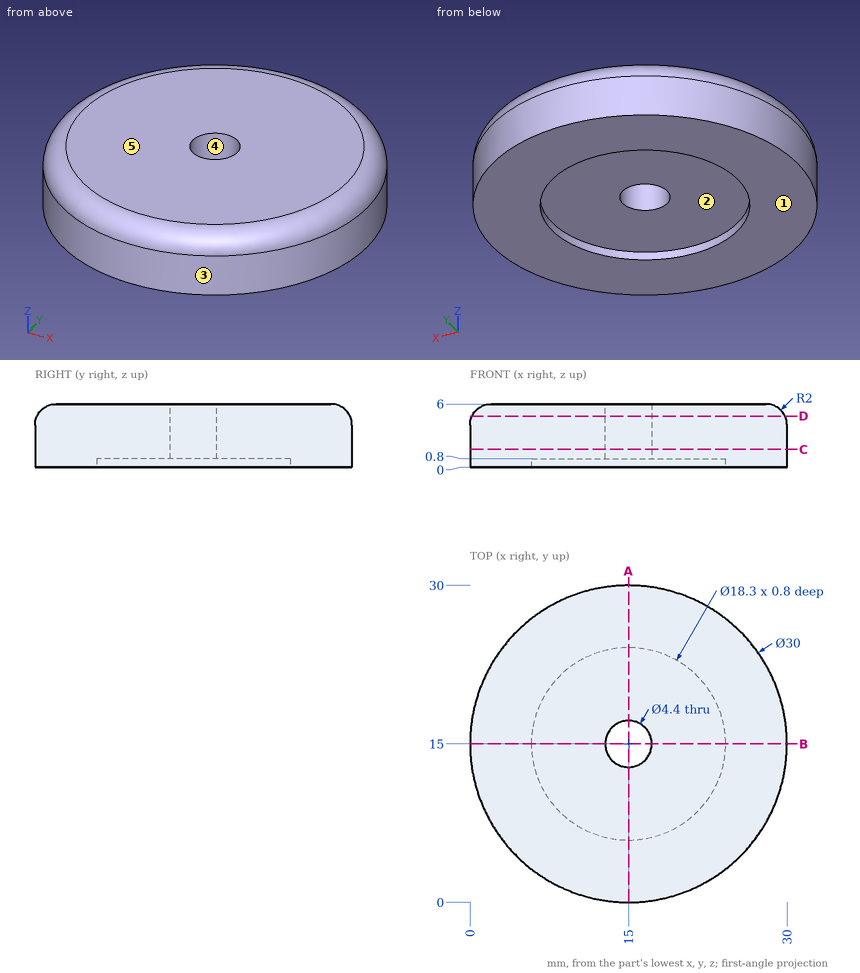
Part print with two shaded views. Sizes in mm from the minimum x, y, z corner. A direction names the side the tool comes from. Round coordinates to 2 decimals unless told otherwise and drop trailing zeros. Order: outer loops, then holes, each group sorted by start corner. A loop starts at its lowest first (then second) coordinate and runs counter-clockwise, first axis right, second up. Notation, with made-up numbers: (69, 21.5) - (111, 21.5) arc R23 cw to (111, 60.5) - close; hole circle Ø8 at (-27, -21). An arc over 180 degrees is marked (long way). Answer in a Markdown table with one row per item. Add a question column.
(1) Probe L1, parallel to Y at x = 15, z = 0.6; L2, parallel to Y at x = 15, z = 2.9; L3, parallel to Z at x = 14, y = 22. List the from-to ranges inside material, lowest first. Write a range as [from, to].
(2) Band-saw the part on A-A on x = 15. List the corners of the cut face in (y, z), and give its area (3 significant figures).
(3) Drop flat-ended pins along their axis: pin 1 Ø2 at (y, z) = (6.5, 2.5) entering from -X; pin 2 Ø5.5 at (x, y) = (15, 15) entering from -Z; pin 3 Ø1 at (y, z) = (15, 5) entering from -X. Give the stop position or say it passes through.
(4) Band-saw the part on C-C on z = 1.7. List the corners of the cut face in (x, y).
(5) Band-saw the part on D-D on z = 4.85. List the corners of the cut face in (x, y).
(6) Mould opens along Y. For the marked faces 3, 4 and 5 say: +Y half, -Y half, draft (parallel to the pull), parting line (faces both ways), or undercut.
(7) 3-axis set-ups, long thin cutter, end or side, ignore diameter. For the marked faces 1 and 2: which of +Z, -Z, +X, -X, +Y, -Y reach the whole face in a straight line?
Data:
| question | item | result |
|---|---|---|
| 1 | L1 | y = [0, 5.85], [24.15, 30] |
| 1 | L2 | y = [0, 12.8], [17.2, 30] |
| 1 | L3 | z = [0.8, 6] |
| 2 | outline | (0, 0) - (5.85, 0) - (5.85, 0.8) - (12.8, 0.8) - (12.8, 6) - (2, 6) arc R2 ccw to (0, 4) - close; (17.2, 0.8) - (24.15, 0.8) - (24.15, 0) - (30, 0) - (30, 4) arc R2 ccw to (28, 6) - (17.2, 6) - close |
| 2 | area | 141 mm^2 |
| 3 | pin 1 | stops at x = 2.01 |
| 3 | pin 2 | stops at z = 0.8 |
| 3 | pin 3 | stops at x = 0.06 |
| 4 | outline | circle Ø30 at (15, 15); hole circle Ø4.4 at (15, 15) |
| 5 | outline | circle Ø29.62 at (15, 15); hole circle Ø4.4 at (15, 15) |
| 6 | face 3 | parting line |
| 6 | face 4 | undercut |
| 6 | face 5 | draft |
| 7 | face 1 | -Z, +X, -X, +Y, -Y |
| 7 | face 2 | -Z |
